```python
from build123d import *

# Parameters (mm, degrees)
SKETCH1_W           = 19.6
SKETCH1_H           = 39.6
BOSS_EXTRUDE1_DEPTH = 39.9
SKETCH2_R           = 2.89
BOSS_EXTRUDE2_DEPTH = 5.08
SKETCH3_W           = 19.6
SKETCH3_H           = 53.6
BOSS_EXTRUDE3_DEPTH = 2.8
SKETCH4_R           = 2.05
CUT_EXTRUDE1_DEPTH  = 59.887689748
FILLET1_R           = 2.54
CUT_EXTRUDE3_START  = -3
CUT_EXTRUDE3_DEPTH  = 3


with BuildPart() as part:
    # Sketch1 → Boss-Extrude1 (new body)
    with BuildSketch(Plane.XY):
        with Locations((9.8, -19.8)):
            Rectangle(SKETCH1_W, SKETCH1_H)
    extrude(amount=BOSS_EXTRUDE1_DEPTH)

    # Sketch2 → Boss-Extrude2 (add)
    with BuildSketch(Plane.XY.offset(39.9)):
        with Locations((9.8, -10)):
            Circle(SKETCH2_R)
    extrude(amount=BOSS_EXTRUDE2_DEPTH)

    # Sketch3 → Boss-Extrude3 (add)
    with BuildSketch(Plane.XY.offset(27.400000064)):
        with Locations((9.8, -19.8)):
            Rectangle(SKETCH3_W, SKETCH3_H)
    extrude(amount=BOSS_EXTRUDE3_DEPTH)

    # Sketch4 → Cut-Extrude1 (cut, through all)
    with BuildSketch(Plane.XY.offset(30.200000064)):
        with Locations((4.8, 4.7)):
            Circle(SKETCH4_R)
        with Locations((14.8, 4.7)):
            Circle(SKETCH4_R)
        with Locations((4.8, -44.3)):
            Circle(SKETCH4_R)
        with Locations((14.8, -44.3)):
            Circle(SKETCH4_R)
    extrude(amount=-CUT_EXTRUDE1_DEPTH, mode=Mode.SUBTRACT)

    # Fillet1
    fillet1_edges = [part.edges().sort_by_distance(p)[0] for p in [
        (19.6, -46.6, 28.800000064),
        (0, 7, 28.800000064),
        (0, -46.6, 28.800000064),
        (19.6, 7, 28.800000064),
    ]]
    fillet(fillet1_edges, radius=FILLET1_R)

    # Sketch5 → Cut-Extrude3 (cut)
    with BuildSketch(Plane.XY.offset(44.98).offset(CUT_EXTRUDE3_START)):
        with BuildLine():
            ThreePointArc((10.518713774, -7.200794664), (10.162213045, -7.132788513), (9.8, -7.11))
            Line((9.8, -7.11), (10.081999776, -7.767741922))
            Line((10.081999776, -7.767741922), (10.518713774, -7.200794664))
        make_face()
        with BuildLine():
            Line((9.518000224, -7.767741922), (9.8, -7.11))
            ThreePointArc((9.8, -7.11), (9.437786955, -7.132788513), (9.081286226, -7.200794664))
            Line((9.081286226, -7.200794664), (9.518000224, -7.767741922))
        make_face()
        with BuildLine():
            Line((8.971719756, -7.908002907), (9.081286226, -7.200794664))
            ThreePointArc((9.081286226, -7.200794664), (8.736120043, -7.312945956), (8.407731882, -7.467473695))
            Line((8.407731882, -7.467473695), (8.971719756, -7.908002907))
        make_face()
        with BuildLine():
            Line((8.477483182, -8.179711763), (8.407731882, -7.467473695))
            ThreePointArc((8.407731882, -7.467473695), (8.101300621, -7.661940886), (7.821658864, -7.893280667))
            Line((7.821658864, -7.893280667), (8.477483182, -8.179711763))
        make_face()
        with BuildLine():
            Line((8.066345204, -8.565796023), (7.821658864, -7.893280667))
            ThreePointArc((7.821658864, -7.893280667), (7.573216728, -8.15784467), (7.359892295, -8.451460563))
            Line((7.359892295, -8.451460563), (8.066345204, -8.565796023))
        make_face()
        with BuildLine():
            Line((7.764139132, -9.041996594), (7.359892295, -8.451460563))
            ThreePointArc((7.359892295, -8.451460563), (7.185049818, -8.769497847), (7.051446668, -9.106940886))
            Line((7.051446668, -9.106940886), (7.764139132, -9.041996594))
        make_face()
        with BuildLine():
            Line((7.589853686, -9.578392042), (7.051446668, -9.106940886))
            ThreePointArc((7.051446668, -9.106940886), (6.961189845, -9.458468001), (6.915702755, -9.818535399))
            Line((6.915702755, -9.818535399), (7.589853686, -9.578392042))
        make_face()
        with BuildLine():
            Line((7.554439861, -10.141278669), (6.915702755, -9.818535399))
            ThreePointArc((6.915702755, -9.818535399), (6.915702755, -10.181464601), (6.961189845, -10.541531999))
            Line((6.961189845, -10.541531999), (7.554439861, -10.141278669))
        make_face()
        with BuildLine():
            Line((7.660122838, -10.695288237), (6.961189845, -10.541531999))
            ThreePointArc((6.961189845, -10.541531999), (7.051446668, -10.893059114), (7.185049818, -11.230502153))
            Line((7.185049818, -11.230502153), (7.660122838, -10.695288237))
        make_face()
        with BuildLine():
            ThreePointArc((11.778341136, -7.893280667), (11.498699379, -7.661940886), (11.192268118, -7.467473695))
            Line((11.192268118, -7.467473695), (11.122516818, -8.179711763))
            Line((11.122516818, -8.179711763), (11.778341136, -7.893280667))
        make_face()
        with BuildLine():
            ThreePointArc((11.192268118, -7.467473695), (10.863879957, -7.312945956), (10.518713774, -7.200794664))
            Line((10.518713774, -7.200794664), (10.628280244, -7.908002907))
            Line((10.628280244, -7.908002907), (11.192268118, -7.467473695))
        make_face()
        with BuildLine():
            ThreePointArc((12.240107705, -8.451460563), (12.026783272, -8.15784467), (11.778341136, -7.893280667))
            Line((11.778341136, -7.893280667), (11.533654796, -8.565796023))
            Line((11.533654796, -8.565796023), (12.240107705, -8.451460563))
        make_face()
        with BuildLine():
            ThreePointArc((12.548553332, -9.106940886), (12.414950182, -8.769497847), (12.240107705, -8.451460563))
            Line((12.240107705, -8.451460563), (11.835860868, -9.041996594))
            Line((11.835860868, -9.041996594), (12.548553332, -9.106940886))
        make_face()
        with BuildLine():
            ThreePointArc((12.684297245, -9.818535399), (12.638810155, -9.458468001), (12.548553332, -9.106940886))
            Line((12.548553332, -9.106940886), (12.010146314, -9.578392042))
            Line((12.010146314, -9.578392042), (12.684297245, -9.818535399))
        make_face()
        with BuildLine():
            ThreePointArc((12.69, -10), (12.688573959, -9.909222906), (12.684297245, -9.818535399))
            Line((12.684297245, -9.818535399), (12.045560139, -10.141278669))
            Line((12.045560139, -10.141278669), (12.638810155, -10.541531999))
            ThreePointArc((12.638810155, -10.541531999), (12.677174078, -10.271973025), (12.69, -10))
        make_face()
        with BuildLine():
            ThreePointArc((12.414950182, -11.230502153), (12.548553332, -10.893059114), (12.638810155, -10.541531999))
            Line((12.638810155, -10.541531999), (11.939877162, -10.695288237))
            Line((11.939877162, -10.695288237), (12.414950182, -11.230502153))
        make_face()
        with BuildLine():
            ThreePointArc((12.026783272, -11.84215533), (12.240107705, -11.548539437), (12.414950182, -11.230502153))
            Line((12.414950182, -11.230502153), (11.699737832, -11.205610289))
            Line((11.699737832, -11.205610289), (12.026783272, -11.84215533))
        make_face()
        with BuildLine():
            ThreePointArc((11.498699379, -12.338059114), (11.778341136, -12.106719333), (12.026783272, -11.84215533))
            Line((12.026783272, -11.84215533), (11.340230988, -11.640179412))
            Line((11.340230988, -11.640179412), (11.498699379, -12.338059114))
        make_face()
        with BuildLine():
            ThreePointArc((10.863879957, -12.687054044), (11.192268118, -12.532526305), (11.498699379, -12.338059114))
            Line((11.498699379, -12.338059114), (10.883945767, -11.97169003))
            Line((10.883945767, -11.97169003), (10.863879957, -12.687054044))
        make_face()
        with BuildLine():
            ThreePointArc((10.162213045, -12.867211487), (10.518713774, -12.799205336), (10.863879957, -12.687054044))
            Line((10.863879957, -12.687054044), (10.359552246, -12.179312113))
            Line((10.359552246, -12.179312113), (10.162213045, -12.867211487))
        make_face()
        with BuildLine():
            Line((9.8, -12.25), (9.437786955, -12.867211487))
            ThreePointArc((9.437786955, -12.867211487), (9.8, -12.89), (10.162213045, -12.867211487))
            Line((10.162213045, -12.867211487), (9.8, -12.25))
        make_face()
        with BuildLine():
            Line((9.240447754, -12.179312113), (8.736120043, -12.687054044))
            ThreePointArc((8.736120043, -12.687054044), (9.081286226, -12.799205336), (9.437786955, -12.867211487))
            Line((9.437786955, -12.867211487), (9.240447754, -12.179312113))
        make_face()
        with BuildLine():
            Line((8.716054233, -11.97169003), (8.101300621, -12.338059114))
            ThreePointArc((8.101300621, -12.338059114), (8.407731882, -12.532526305), (8.736120043, -12.687054044))
            Line((8.736120043, -12.687054044), (8.716054233, -11.97169003))
        make_face()
        with BuildLine():
            Line((8.259769012, -11.640179412), (7.573216728, -11.84215533))
            ThreePointArc((7.573216728, -11.84215533), (7.821658864, -12.106719333), (8.101300621, -12.338059114))
            Line((8.101300621, -12.338059114), (8.259769012, -11.640179412))
        make_face()
        with BuildLine():
            Line((7.900262168, -11.205610289), (7.185049818, -11.230502153))
            ThreePointArc((7.185049818, -11.230502153), (7.359892295, -11.548539437), (7.573216728, -11.84215533))
            Line((7.573216728, -11.84215533), (7.900262168, -11.205610289))
        make_face()
    extrude(amount=CUT_EXTRUDE3_DEPTH, mode=Mode.SUBTRACT)


solid = part.part
```
Geometry check sheet. Reference: the model listing, model coordinates, mm. A direction names the side the tool comes from. Give positions to 0.01 mm unless a question says otherwise; leave off trailing zeros. Order: outer loops, then holes, each group sorted by start corner. A loop starts at its lowest first (then second) coordinate and runs counter-clockwise, first axis right, second up. Notation, with made-up numbers: (24, -14) - (67, -14) arc R31 cw to (67, 18) - close; hole circle Ø8 at (26, 20.25). An arc over 180 degrees is marked (long way). Write item = value, one per line. Start each with the question number.
1) Section check D-D (x = 1.5). Enter the section's corners in (y, z), then the cut area to 3 significant figures.
2) Section check B-B (y = -3.5). Enter the section's corners in (x, z).
3) Gauge pin test, flat ends, axial feed: pin 1 Ø10 at (x, y) = (14, -2) entering from +Z; pin 2 Ø5.5 at (x, y) = (4.8, -44.3) entering from +Z; pin 3 Ø3 at (x, z) = (10.5, 36.5) entering from -Y. Record the tip position at first contact, or that the pin passes through.
4) Section check A-A (x = 4.8). Enter the section's corners in (y, z).
5) Access from +Z, -Z, +X, -X, +Y, -Y to the whole of each face (thin tool, end or side, straight path). Record for faces 1 (the flat face through (10, 0, 14)), 2 (the flat face through (10, -39.6, 35)), 3 (the flat face through (10, -39.6, 14)), 4 (the cylindrical face through (12.47, -11.11, 40.93)).
6) Scan lines: L1, parallel to Y at x = 14.8, z = 29.6; L2, parallel to X at y = 4, z = 29; L3, parallel to Z at x = 13.25, y = -24.5. Record each from-to range of solid material in increasing order.
7) Draft check along Y on faces 5 (the flat face through (10, -42, 30.2)), 6 (the cylindrical face through (3.3, 6.1, 28.8)), 7 (the cylindrical face through (18.836, -45.876, 28.82)). Enter one of: released by +Y, released by -Y, zero draft, split by the parting line, or undercut.
8) Section check C-C (z = 26.5). Enter the section's corners in (x, y), then the cut area to 3 significant figures.
Geometry check:
q1.outline = (-46.38, 27.4) - (-39.6, 27.4) - (-39.6, 0) - (0, 0) - (0, 27.4) - (6.78, 27.4) - (6.78, 30.2) - (0, 30.2) - (0, 39.9) - (-39.6, 39.9) - (-39.6, 30.2) - (-46.38, 30.2) - close
q1.area = 1,620 mm2
q2.outline = (0, 0) - (19.6, 0) - (19.6, 39.9) - (0, 39.9) - close
q3.pin_1 = 39.9
q3.pin_2 = 30.2
q3.pin_3 = -39.6
q4.outline = (-46.6, 27.4) - (-46.35, 27.4) - (-46.35, 30.2) - (-46.6, 30.2) - close; (-42.25, 27.4) - (-39.6, 27.4) - (-39.6, 0) - (0, 0) - (0, 27.4) - (2.65, 27.4) - (2.65, 30.2) - (0, 30.2) - (0, 39.9) - (-39.6, 39.9) - (-39.6, 30.2) - (-42.25, 30.2) - close; (6.75, 27.4) - (7, 27.4) - (7, 30.2) - (6.75, 30.2) - close
q5.face_1 = -Z, +X, -X, +Y
q5.face_2 = +Z, +X, -X, -Y
q5.face_3 = -Z, +X, -X, -Y
q5.face_4 = +Z
q6.L1 = -46.6 to -46.35, -42.25 to 2.65, 6.75 to 7
q6.L2 = 0 to 2.87, 6.73 to 12.87, 16.73 to 19.6
q6.L3 = 0 to 39.9
q7.face_5 = zero draft
q7.face_6 = undercut
q7.face_7 = released by -Y
q8.outline = (0, -39.6) - (19.6, -39.6) - (19.6, 0) - (0, 0) - close
q8.area = 776 mm2
